Geometry: final body of the model. Coordinates: model frame, mm. A direction names the side the tool comes from. Give positions to 0.01 mm unless a question says otherwise; leave off trailing zeros. Loops run counter-clockwise (first coordinate to the right, second up) from the corner with the lowest first, then second, coordinate; pieces in that order, holes last.
from build123d import *

# Parameters (mm, degrees)
SKETCH1_W                                           = 78
SKETCH1_H                                           = 45
SKETCH1_R                                           = 1.65
BOSS_EXTRUDE1_DEPTH                                 = 2
BOSS_EXTRUDE2_START                                 = 5
SKETCH1_3_W                                         = 10
SKETCH1_3_H                                         = 45
SKETCH1_3_R                                         = 1.65
BOSS_EXTRUDE2_DEPTH                                 = 5
BOSS_EXTRUDE3_START                                 = 19
SKETCH1_4_W                                         = 10
SKETCH1_4_H                                         = 45
SKETCH1_4_R                                         = 1.65
BOSS_EXTRUDE3_DEPTH                                 = 19
CHAMFER2_SIZE2                                      = 5
CHAMFER2_SIZE                                       = 7
CUT_EXTRUDE1_DEPTH                                  = 63
CSK_FOR_M3_COUNTERSUNK_FLAT_HEAD_SCREW1_D           = 3.6
CSK_FOR_M3_COUNTERSUNK_FLAT_HEAD_SCREW1_CSINK_D     = 6.3
CSK_FOR_M3_COUNTERSUNK_FLAT_HEAD_SCREW1_CSINK_ANGLE = 90
CSK_FOR_M3_COUNTERSUNK_FLAT_HEAD_SCREW2_D           = 3.6
CSK_FOR_M3_COUNTERSUNK_FLAT_HEAD_SCREW2_CSINK_D     = 6.3
CSK_FOR_M3_COUNTERSUNK_FLAT_HEAD_SCREW2_CSINK_ANGLE = 90


with BuildPart() as part:
    # Sketch1 → Boss-Extrude1 (new body)
    with BuildSketch(Plane.XY):
        Rectangle(SKETCH1_W, SKETCH1_H)
        with Locations((34, 0)):
            Circle(SKETCH1_R, mode=Mode.SUBTRACT)
        with Locations((-34, -18)):
            Circle(SKETCH1_R, mode=Mode.SUBTRACT)
        with Locations((-34, 18)):
            Circle(SKETCH1_R, mode=Mode.SUBTRACT)
    extrude(amount=-BOSS_EXTRUDE1_DEPTH)

    # Sketch1<3> → Boss-Extrude2 (add)
    # profile 1 of 2: a face of its own
    with BuildSketch(Plane.XY.offset(BOSS_EXTRUDE2_START)):
        with Locations((-34, 0)):
            Rectangle(SKETCH1_3_W, SKETCH1_3_H)
        with Locations((-34, -18)):
            Circle(SKETCH1_3_R, mode=Mode.SUBTRACT)
        with Locations((-34, 18)):
            Circle(SKETCH1_3_R, mode=Mode.SUBTRACT)
    # profile 2 of 2: a face of its own
    with BuildSketch(Plane.XY.offset(BOSS_EXTRUDE2_START)):
        with Locations((34, 0)):
            Rectangle(SKETCH1_3_W, SKETCH1_3_H)
        with Locations((34, 0)):
            Circle(SKETCH1_3_R, mode=Mode.SUBTRACT)
    extrude(amount=-BOSS_EXTRUDE2_DEPTH)

    # Sketch1<4> → Boss-Extrude3 (add)
    with BuildSketch(Plane.XY.offset(BOSS_EXTRUDE3_START)):
        with Locations((-34, 0)):
            Rectangle(SKETCH1_4_W, SKETCH1_4_H)
        with Locations((-34, -18)):
            Circle(SKETCH1_4_R, mode=Mode.SUBTRACT)
        with Locations((-34, 18)):
            Circle(SKETCH1_4_R, mode=Mode.SUBTRACT)
    extrude(amount=-BOSS_EXTRUDE3_DEPTH)

    # Chamfer2
    chamfer2_edges = [part.edges().sort_by_distance(p)[0] for p in [
        (29, 0, 0),
    ]]
    chamfer2_side = [part.faces().sort_by_distance(p)[0] for p in [
        (28.9, 0, 0),
    ]]
    chamfer(chamfer2_edges, length=CHAMFER2_SIZE - 0.0001, length2=CHAMFER2_SIZE2 - 0.0001, reference=chamfer2_side[0])  # a hair under: the kernel refuses the full size

    # Sketch2 → Cut-Extrude1 (cut)
    with BuildSketch(Plane.XZ.offset(22.5)):
        Polygon((22.640930107, -2), (29, 2.542192781), (39, 2.542192781), (39, -2), align=None)
    extrude(amount=-CUT_EXTRUDE1_DEPTH, mode=Mode.SUBTRACT)

    # CSK for M3 Countersunk Flat Head Screw1 (through all)
    with Locations(Plane(origin=(0, 0, 2.542192781), x_dir=(-1, 0, 0), z_dir=(0, 0, -1))):
        with Locations((-34, 0)):
            CounterSinkHole(CSK_FOR_M3_COUNTERSUNK_FLAT_HEAD_SCREW1_D / 2, CSK_FOR_M3_COUNTERSUNK_FLAT_HEAD_SCREW1_CSINK_D / 2, counter_sink_angle=CSK_FOR_M3_COUNTERSUNK_FLAT_HEAD_SCREW1_CSINK_ANGLE)

    # CSK for M3 Countersunk Flat Head Screw2 (through all)
    with Locations(Plane(origin=(0, 0, -2), x_dir=(-1, 0, 0), z_dir=(0, 0, -1))):
        with Locations((34, -18), (34, 18)):
            CounterSinkHole(CSK_FOR_M3_COUNTERSUNK_FLAT_HEAD_SCREW2_D / 2, CSK_FOR_M3_COUNTERSUNK_FLAT_HEAD_SCREW2_CSINK_D / 2, counter_sink_angle=CSK_FOR_M3_COUNTERSUNK_FLAT_HEAD_SCREW2_CSINK_ANGLE)


solid = part.part
Item 1: Section query B-B on x = -34. Return loops of the section in (y, z).
Values follow:
outline: (-22.5, -2) - (-21.15, -2) - (-19.8, -0.65) - (-19.8, 19) - (-22.5, 19) - close; (-16.2, -0.65) - (-14.85, -2) - (14.85, -2) - (16.2, -0.65) - (16.2, 19) - (-16.2, 19) - close; (19.8, -0.65) - (21.15, -2) - (22.5, -2) - (22.5, 19) - (19.8, 19) - close
Item 2: Pin query (flat end, axial travel): pin 1 (8 mm diameter, centred on x = 33.5, y = 4.5, fed in from +Z); pin 2 (1 mm diameter, centred on x = 9.5, y = 4.5, fed in from +Z); pin 3 (6 mm diameter, centred on y = -9, z = 14, fed in from +X). Return the tip coordinate at first contact, or that it passes through.
Values follow:
pin 1: stops at z = 5
pin 2: stops at z = 0
pin 3: stops at x = -29
Item 3: Draft query along X for faces 5 (the face through (25.78, -0.32, 0.24)), 6 (the face through (-33.032, 19.518, 9.313)), 7 (the face through (-4, 0, 0)), 8 (the face through (-18, -22.5, -1)). Return one class per face: +X half, -X half, draft (parallel to the pull), parting line (faces both ways), or undercut.
Values follow:
face 5: +X half
face 6: undercut
face 7: undercut
face 8: draft
Item 4: Section query C-C on x = 34. Return loops of the section in (y, z).
Values follow:
outline: (-22.5, 2.54) - (-3.15, 2.54) - (-1.8, 3.89) - (-1.8, 5) - (-22.5, 5) - close; (1.8, 3.89) - (3.15, 2.54) - (22.5, 2.54) - (22.5, 5) - (1.8, 5) - close
Item 5: Set-up query: faces 1 (the face through (-34, 0, 19)), 2 (the face through (37.3, -0.3, 2.542)), 3 (the face through (-29, 0, 10)), 4 (the face through (36, 0, 5)). Return all of +Z, -Z, +X, -X, +Y, -Y with unobstructed straight access to the full face (end or side cutting, diameter ignored); none if empty.
Values follow:
face 1: +Z, +X, -X, +Y, -Y
face 2: -Z, +X, +Y, -Y
face 3: +Z, +Y, -Y
face 4: +Z, +X, +Y, -Y
Item 6: Ray query, probe 1 along Y at (x, z) = (-34, 8.75); probe 2 along Y at (x, z) = (34, 4.5); probe 3 along X at (y, z) = (19, 3.25). Return the intervals inside material, ascending.
Values follow:
probe 1: y = -22.5 to -19.8, -16.2 to 16.2, 19.8 to 22.5
probe 2: y = -22.5 to -1.8, 1.8 to 22.5
probe 3: x = -39 to -35.5, -32.5 to -29, 26.55 to 39
